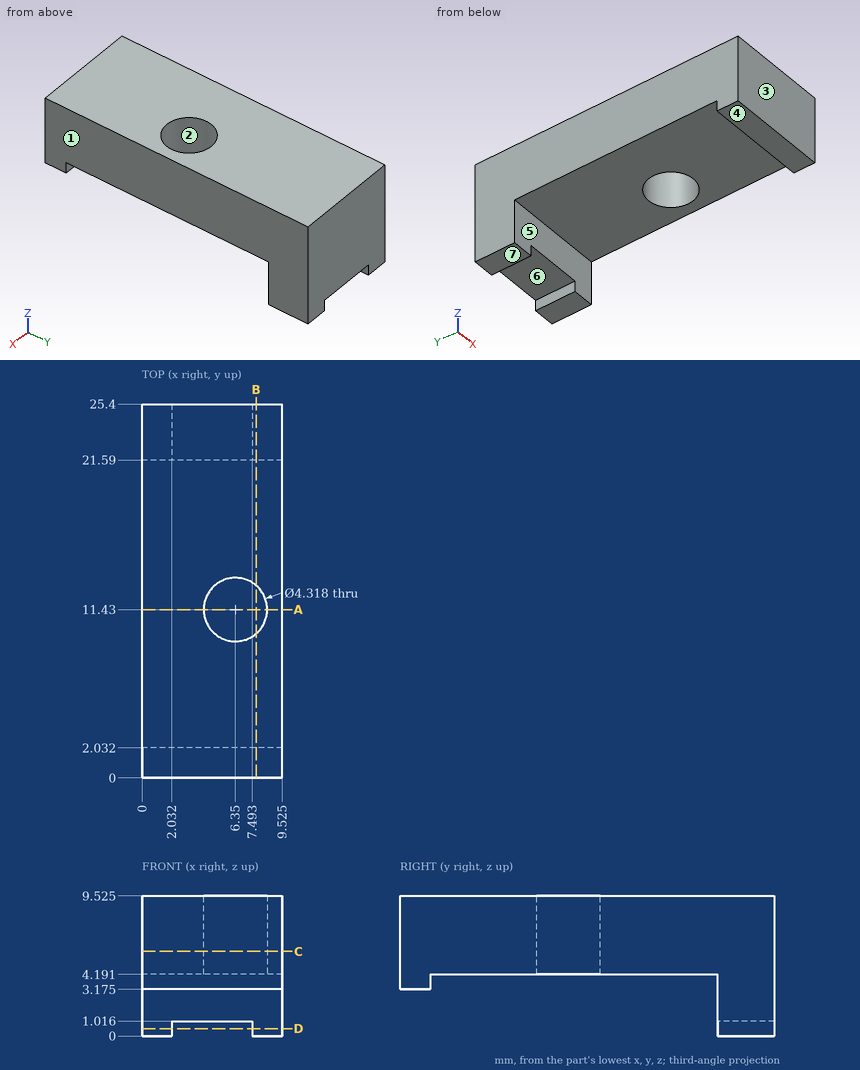
Geometry: see drawing. Coordinates: mm, zero at the bounding-box minimum. A direction names the side the tool comes from. Round coordinates to 2 decimals unless told otherwise and drop trailing zeros. Loops run counter-clockwise (first coordinate to the right, second up) from the corner with the lowest first, then second, coordinate; pieces in that order, holes last. Notation, with made-up numbers: (73.5, 62) - (98.5, 62) arc R6 ccw to (98.5, 71) - close; hole circle Ø9 at (-6.5, 64.25). An arc over 180 degrees is marked (long way). Write item = value, one per line. Start each with the question number.
(1) Section query C-C, the plane z = 5.75. Output: boundary loops of the cut face in (x, y) (3 decimals), plus the area to 3 significant figures.
(2) Section query A-A, the plane y = 11.43. Output: boundary loops of the cut face in (x, z) (3 decimals), plus the area to 3 significant figures.
(3) Section query B-B, the plane x = 7.75. Output: boundary loops of the cut face in (y, z) (3 decimals), plus the area to 3 significant figures.
(4) Pin query (flat end, axial travel): pin 1 (4 mm diameter, centred on x = 5, z = 4.5, fed in from -Y); pin 2 (0.6 mm diameter, centred on x = 3.5, y = 1, fed in from -Z) (3 decimals); pin 3 (3 mm diameter, centred on x = 5, y = 13.5, fed in from -Z); pin 4 (1.1 mm diameter, centred on x = 3.5, y = 23.5, fed in from -Z). Return the tip coordinate at first contact, or that it passes through.
(5) Ray query, line 1 along Y through (x, z) = (4.5, 3.5); line 2 along Y through (x, z) = (6.35, 7.6); line 3 along Z through (x, y) = (8, 16.75) (3 decimals). Return the intervals inside material, ascending. Write a range as from..to.
(6) Pull-direction query (Y, two-part tool) for the marked faces 1, 2 and 3; classes: +Y half, -Y half, draft (parallel to the pull), parting line (faces both ways), or undercut.
(7) Section query D-D, the plane z = 0.5. Output: boundary loops of the cut face in (x, y) (3 decimals), plus the area to 3 significant figures.
(8) Set-up query: the marked faces 4, 5, 6 and 7. Return all of +Z, -Z, +X, -X, +Y, -Y with unobstructed straight access to the full face (end or side cutting, diameter ignored); none if empty.
Conclusion:
q1.outline = (0, 0) - (9.525, 0) - (9.525, 25.4) - (0, 25.4) - close; hole circle Ø4.318 at (6.35, 11.43)
q1.area = 227 mm2
q2.outline = (0, 4.191) - (4.191, 4.191) - (4.191, 9.525) - (0, 9.525) - close; (8.509, 4.191) - (9.525, 4.191) - (9.525, 9.525) - (8.509, 9.525) - close
q2.area = 27.8 mm2
q3.outline = (0, 3.175) - (2.032, 3.175) - (2.032, 4.191) - (9.786, 4.191) - (9.786, 9.525) - (0, 9.525) - close; (13.074, 4.191) - (21.59, 4.191) - (21.59, 0) - (25.4, 0) - (25.4, 9.525) - (13.074, 9.525) - close
q3.area = 136 mm2
q4.pin_1 = 0
q4.pin_2 = 3.175
q4.pin_3 = 4.19
q4.pin_4 = 1.02
q5.line_1 = 0..2.03, 21.59..25.4
q5.line_2 = 0..9.27, 13.59..25.4
q5.line_3 = 4.191..9.525
q6.face_1 = draft
q6.face_2 = undercut
q6.face_3 = -Y half
q7.outline = (0, 21.59) - (2.032, 21.59) - (2.032, 25.4) - (0, 25.4) - close; (7.493, 21.59) - (9.525, 21.59) - (9.525, 25.4) - (7.493, 25.4) - close
q7.area = 15.5 mm2
q8.face_4 = -Z, +X, -X, -Y
q8.face_5 = -Z, +X, -X
q8.face_6 = -Z, +Y, -Y
q8.face_7 = -Z, +X, -X, +Y, -Y
